Work out the finished part from the listing and answer in its coordinate system (mm). A direction names the side the tool comes from. Coordinates: 2 decimals unless noted, no trailing zeros. Write each loop counter-clockwise with the first axis right and the second up, starting at its lowest first coordinate (ties: lowest second). Pieces come first, ordered by that corner, then holes. Notation, with made-up numbers: (7.25, 6) - (46.25, 6) arc R17 ccw to (46.25, 17) - close; hole circle Ø6 at (18.25, -15.5). An arc over 180 degrees is marked (long way). Answer as a JSON object with one key per item and string values. Group by question number.
from build123d import *

# Parameters (mm, degrees)
F0_R         = 4.275
F2_R         = 4.925
F4_R         = 4.95
F8_R         = 1.525
F9_DEPTH     = 3.57
F10_R        = 1.3
F11_DEPTH    = 0.83
F13_DEPTH    = 0.46
F14_S5_R     = 1.3
F14_T6_DEPTH = 4


# Not quite as in the source:
# - a fillet or chamfer that OpenCascade refuses, or shapes differently, is made with other operations: its cross-section is extruded or revolved along the edge and cut away or added


with BuildPart() as f6:
    # F0 (on Top) → F6 section 0
    with BuildSketch(Plane.XY):
        Circle(F0_R)
    # F2 (on offset) → F6 section 1
    with BuildSketch(Plane.XY.offset(0.83)):
        Circle(F2_R)
    loft()

    # F2 (on offset) → F7 section 0
    with BuildSketch(Plane.XY.offset(0.83)):
        Circle(F2_R)
    # F4 (on offset) → F7 section 1
    with BuildSketch(Plane.XY.offset(4.4)):
        Circle(F4_R)
    loft()

    # F8 (on face) → F9 (cut, through all)
    with BuildSketch(Plane.XY.offset(4.4)):
        Circle(F8_R)
    extrude(amount=-F9_DEPTH, mode=Mode.SUBTRACT)

    # F10 (on face) → F11 (cut, through all)
    with BuildSketch(Plane(origin=(0, 0, 0), x_dir=(1, 0, 0), z_dir=(0, 0, -1))):
        Circle(F10_R)
    extrude(amount=-F11_DEPTH, mode=Mode.SUBTRACT)

    # F12 (on face) → F13 (cut)
    with BuildSketch(Plane(origin=(0, 0, 0), x_dir=(1, 0, 0), z_dir=(0, 0, -1))):
        Polygon((-0.6, -5), (0, -5), (0.6, -5), (0.6, 0), (0, 0), (-0.6, 0), align=None)
    extrude(amount=-F13_DEPTH, mode=Mode.SUBTRACT)

    # F14: chamfer of 0.5 on 1 edges, made by hand


with BuildPart() as f14_tool2:
    # F14_s3 → F14_t4 (revolve)
    with BuildSketch(Plane.XZ):
        Polygon((1.525, 1.33), (1.025, 0.83), (1.525, 0.83), align=None)
    revolve(axis=Axis((0, 0, 0.83), (0, 0, 1)))

    # F14_s5 → F14_t6 (cut, symmetric)
    with BuildSketch(Plane.XY.offset(1.1)):
        Circle(F14_S5_R)
    extrude(amount=F14_T6_DEPTH, both=True, mode=Mode.SUBTRACT)


with BuildPart() as f6_1:
    add(f6.part)

    # F14_t1: union F14_tool2
    add(f14_tool2.part)


solid = f6_1.part
Q1. For a pull along X with two mould halves and no side action, classify faces 1 (the face through (0, -2, 0)), 2 (the face through (4.71, 1.48, 2.64)), 3 (the face through (0.6, -1.153, 0.56)) as +X half, -X half, draft (parallel to the pull), parting line (faces both ways), or undercut.
Q2. Consider L1, parallel to X at y = 0, z = 0.55; L2, parallel to X at y = 0, z = 0.3. Determine where each line is inside the solid, lowest interval first. Write a range as from..to.
Q3. A tool of negligible diameter and unlimited length cuts with its end or side. For faces 4 (the face through (2.02, -3.89, 0.14)), 5 (the face through (0, 3, 0.46)), 6 (the face through (-1.524, 0.067, 2.886)), from which of +Z, -Z, +X, -X, +Y, -Y can it reach the whole face along a straight path? Write none if from no direction.
Q4. Flat-ended cylindrical pins translate along their axes: pin 1 Ø0.5 at (y, z) = (2.5, 0) entering from -X; pin 2 Ø1.5 at (x, z) = (-0.5, 2) entering from +Y; pin 3 Ø2.5 at (x, y) = (0, 0) entering from -Z; pin 4 Ø1 at (x, y) = (0, 3.5) entering from -Z. Find the tip coordinate at first contact, or state that the pin passes through.
Q5. Section A-A on z = 2.6 is taken. Determine the outline of the cut face in (x, y) (3 decimals).
Numbers:
{
 "1": {"face 1": "draft", "face 2": "parting line", "face 3": "undercut"},
 "2": {"L1": "x = -4.71..-1.3, 1.3..4.71", "L2": "x = -4.51..-1.3, 1.3..4.51"},
 "3": {"face 4": "-Z", "face 5": "-Z, +Y", "face 6": "+Z"},
 "4": {"pin 1": "stops at x = -3.76", "pin 2": "stops at y = 4.94", "pin 3": "passes through", "pin 4": "stops at z = 0.46"},
 "5": {"outline": "circle Ø9.875 at (0, 0); hole circle Ø3.05 at (0, 0)"}
}
